```python
from build123d import *

# Parameters (mm, degrees)
SKETCH1_R           = 2.5
SKETCH1_R_2         = 1.6
BOSS_EXTRUDE1_DEPTH = 3
SKETCH2_W           = 2
SKETCH2_H           = 2
CUT_EXTRUDE1_DEPTH  = 117.880152293


with BuildPart() as part:
    # Sketch1 → Boss-Extrude1 (new body)
    with BuildSketch(Plane(origin=(0, 0, 0), x_dir=(1, 0, 0), z_dir=(0, 1, 0))):
        with BuildLine():
            Line((-64.6, -70.6), (64.6, -70.6))
            ThreePointArc((64.6, -70.6), (68.842640687, -68.842640687), (70.6, -64.6))
            Line((70.6, -64.6), (70.6, 64.6))
            ThreePointArc((70.6, 64.6), (69.163190657, 68.495804286), (65.540902989, 70.525765905))
            ThreePointArc((65.540902989, 70.525765905), (64.340790015, 70.792848887), (63.182522555, 71.205184867))
            Line((63.182522555, 71.205184867), (13.781138102, 92.296857547))
            ThreePointArc((13.781138102, 92.296857547), (11.858510235, 92.897157125), (9.854586018, 93.1))
            Line((9.854586018, 93.1), (6, 93.1))
            Line((6, 93.1), (6, 73.1))
            Line((6, 73.1), (-6, 73.1))
            Line((-6, 73.1), (-6, 93.1))
            Line((-6, 93.1), (-9.854586018, 93.1))
            ThreePointArc((-9.854586018, 93.1), (-11.858510235, 92.897157125), (-13.781138102, 92.296857547))
            Line((-13.781138102, 92.296857547), (-63.182522555, 71.205184867))
            ThreePointArc((-63.182522555, 71.205184867), (-64.340790015, 70.792848887), (-65.540902989, 70.525765905))
            ThreePointArc((-65.540902989, 70.525765905), (-69.163190657, 68.495804286), (-70.6, 64.6))
            Line((-70.6, 64.6), (-70.6, -64.6))
            ThreePointArc((-70.6, -64.6), (-68.842640687, -68.842640687), (-64.6, -70.6))
        make_face()
        with Locations(Location((64.6, -64.6, 0), (0, 0, 270))):
            Circle(SKETCH1_R, mode=Mode.SUBTRACT)
        with Locations(Location((48.6, -64.6, 0), (0, 0, 270))):
            Circle(SKETCH1_R, mode=Mode.SUBTRACT)
        with Locations(Location((-55.87, 64.6, 0), (0, 0, 270))):
            Circle(SKETCH1_R_2, mode=Mode.SUBTRACT)
        with Locations(Location((55.87, -64.6, 0), (0, 0, 270))):
            Circle(SKETCH1_R_2, mode=Mode.SUBTRACT)
        with Locations(Location((-48.6, 64.6, 0), (0, 0, 270))):
            Circle(SKETCH1_R, mode=Mode.SUBTRACT)
        with Locations(Location((55.87, 64.6, 0), (0, 0, 270))):
            Circle(SKETCH1_R_2, mode=Mode.SUBTRACT)
        with Locations(Location((48.6, 64.6, 0), (0, 0, 270))):
            Circle(SKETCH1_R, mode=Mode.SUBTRACT)
        with Locations(Location((64.6, 64.6, 0), (0, 0, 270))):
            Circle(SKETCH1_R, mode=Mode.SUBTRACT)
        with Locations(Location((-55.87, -64.6, 0), (0, 0, 270))):
            Circle(SKETCH1_R_2, mode=Mode.SUBTRACT)
        with Locations(Location((-48.6, -64.6, 0), (0, 0, 270))):
            Circle(SKETCH1_R, mode=Mode.SUBTRACT)
        with Locations(Location((-64.6, -64.6, 0), (0, 0, 270))):
            Circle(SKETCH1_R, mode=Mode.SUBTRACT)
        with Locations(Location((-64.6, 64.6, 0), (0, 0, 270))):
            Circle(SKETCH1_R, mode=Mode.SUBTRACT)
        with BuildLine():
            ThreePointArc((-41, 54), (-50.192388155, 50.192388155), (-54, 41))
            Line((-54, 41), (-54, -41))
            ThreePointArc((-54, -41), (-50.192388155, -50.192388155), (-41, -54))
            Line((-41, -54), (41, -54))
            ThreePointArc((41, -54), (50.192388155, -50.192388155), (54, -41))
            Line((54, -41), (54, 41))
            ThreePointArc((54, 41), (50.192388155, 50.192388155), (41, 54))
            Line((41, 54), (-41, 54))
        make_face(mode=Mode.SUBTRACT)
    extrude(amount=BOSS_EXTRUDE1_DEPTH)

    # Sketch2 → Cut-Extrude1 (cut, through all)
    with BuildSketch(Plane(origin=(0, 3, 0), x_dir=(1, 0, 0), z_dir=(0, 1, 0))):
        with Locations((-7, 92.1)):
            Rectangle(SKETCH2_W, SKETCH2_H)
        with Locations((7, 92.1)):
            Rectangle(SKETCH2_W, SKETCH2_H)
        with Locations((-7, -55)):
            Rectangle(SKETCH2_W, SKETCH2_H)
        with Locations((7, -55)):
            Rectangle(SKETCH2_W, SKETCH2_H)
    extrude(amount=-CUT_EXTRUDE1_DEPTH, mode=Mode.SUBTRACT)


solid = part.part
```
Geometry: final body of the model. Coordinates: model frame, mm. A direction names the side the tool comes from. Coordinates: 2 decimals unless noted, no trailing zeros. Order: outer loops, then holes, each group sorted by start corner. A loop starts at its lowest first (then second) coordinate and runs counter-clockwise, first axis right, second up. Notation, with made-up numbers: (-19, 17) - (40, 17) arc R15 ccw to (40, 28) - close; hole circle Ø9 at (54.5, 82.5). An arc over 180 degrees is marked (long way). Write each question's results on one line, items separated by ' | '.
(1) Section query B-B, the plane x = -48.6. Return the cut outline in (y, z), plus the area to 3 significant figures.
Values found:
outline: (0, -77.43) - (3, -77.43) - (3, -67.1) - (0, -67.1) - close; (0, -62.1) - (3, -62.1) - (3, -51.55) - (0, -51.55) - close; (0, 51.55) - (3, 51.55) - (3, 62.1) - (0, 62.1) - close; (0, 67.1) - (3, 67.1) - (3, 70.6) - (0, 70.6) - close | area: 105 mm²
(2) Section query C-C, the plane y = 1.2. Count the separate pieces of the cut face and the enclosed holes in it, plus the area to 3 significant figures.
Values found:
separate pieces: 1 | enclosed holes: 13 | area: 9,660 mm²
(3) First-contact query: pin 1 Ø1.5 at (y, z) = (1.5, -82.5) entering from -X; pin 2 Ø1.5 at (x, y) = (26.5, 2) entering from -Z; pin 3 Ø1 at (x, y) = (51.5, 1) entering from -Z. Flat tips, straight axial feed; report the tip coordinate or a pass-through.
Values found:
pin 1: stops at x = -38.48 | pin 2: stops at z = -87.19 | pin 3: stops at z = -76.41
(4) Set-up query: faces 1 (the face through (-1, 0, -67)), 2 (the face through (50.091, 1.479, 50.293)). Return all of +Z, -Z, +X, -X, +Y, -Y with unobstructed straight access to the full face (end or side cutting, diameter ignored); none if empty.
Values found:
face 1: +Z, -Z, +X, -X, -Y | face 2: +Y, -Y
(5) Line query: line 1 (X direction, y = 2.1, z = 15); line 2 (Z direction, x = -7, y = 1.95); line 3 (Z direction, x = 10, y = 1.75). Output: solid intervals per line, ascending. Write a range as [from, to].
Values found:
line 1: x = [-70.6, -54], [54, 70.6] | line 2: z = [-91.1, -54], [56, 70.6] | line 3: z = [-93.1, -54], [54, 70.6]
(6) Mould query, pull axis X, two halves, no side actions, for faces 3 (the face through (-1, 3, -67)), 4 (the face through (46.16, 1.48, -65.14)), 5 (the face through (69.2, 1.48, -68.45)). Classes: +X half, -X half, draft (parallel to the pull), parting line (faces both ways), or undercut.
Values found:
face 3: draft | face 4: undercut | face 5: +X half
(7) Section query A-A, the plane z = 34. Return the cut outline in (x, y).
Values found:
outline: (-70.6, 0) - (-54, 0) - (-54, 3) - (-70.6, 3) - close; (54, 0) - (70.6, 0) - (70.6, 3) - (54, 3) - close
